```python
from build123d import *

# Parameters (mm, degrees)
SKETCH1_R               = 5.5
BOSS_EXTRUDE1_DEPTH     = 6
CUT_EXTRUDE1_DEPTH      = 3
CUT_EXTRUDE1_DEPTH_BACK = 3
SKETCH3_W               = 5
SKETCH3_H               = 0.446225232


with BuildPart() as part:
    # Sketch1 → Boss-Extrude1 (new body)
    with BuildSketch(Plane(origin=(0, 0, 0), x_dir=(1, 0, 0), z_dir=(0, 1, 0))):
        with Locations(Location((0, 0, 0), (0, 0, 270))):
            Circle(SKETCH1_R)
    extrude(amount=BOSS_EXTRUDE1_DEPTH)

    # Sketch3 → Cut-Extrude1 (cut, two sides: drawn at the far end of the back side and taken through both)
    with BuildSketch(Plane(origin=(0, 3, 3), x_dir=(1, 0, 0), z_dir=(0, 0.7071067811865464, 0.7071067811865488)).offset(-CUT_EXTRUDE1_DEPTH_BACK)):
        with Locations((0.083557951, 4.409395003)):
            Rectangle(SKETCH3_W, SKETCH3_H)
    extrude(amount=CUT_EXTRUDE1_DEPTH + CUT_EXTRUDE1_DEPTH_BACK, mode=Mode.SUBTRACT)


solid = part.part
```
Check sheet for the modelled part. Datum: model origin and axes. Units: mm. A direction names the side the tool comes from. Round coordinates to 2 decimals unless told otherwise and drop trailing zeros. Order: outer loops, then holes, each group sorted by start corner. A loop starts at its lowest first (then second) coordinate and runs counter-clockwise, first axis right, second up. Notation, with made-up numbers: M 50,45 L 65,45 A11 ccw 65,52 Z; hole C 62,-20 d2. An arc over 180 degrees is marked long. Answer in a Markdown table with one row per item.
(1) Gauge pin test, flat ends, axial feed: pin 1 (1.7 mm diameter, centred on y = 5, z = -1.5, fed in from +X); pin 2 (1 mm diameter, centred on x = -2, y = 3.5, fed in from +Z); pin 3 (1.5 mm diameter, centred on y = 5.5, z = 1.5, fed in from +X); pin 4 (1 mm diameter, centred on x = 0.5, z = -2, fed in from -Y). Record the tip position at first contact, or that the pin passes through.
Findings:
| item | result |
|---|---|
| pin 1 | stops at x = 5.46 |
| pin 2 | stops at z = 5.29 |
| pin 3 | stops at x = 5.45 |
| pin 4 | stops at y = 0 |
(2) Draft check along Y on faces 3 (the flat face through (2.584, 5.1, -1.2)), 4 (the cylindrical face through (-5.37, 2.96, -1.19)), 5 (the flat face through (0, 0, 0)). Enter one of: +Y half, -Y half, draft (parallel to the pull), parting line (faces both ways), or undercut.
Findings:
| item | result |
|---|---|
| face 3 | undercut |
| face 4 | draft |
| face 5 | -Y half |
(3) Section check C-C on y = 3.4. Record the boundary of the cut face in (x, z).
Findings:
| item | result |
|---|---|
| outline | C 0,0 d11 |
(4) Material ranges on line 1 along Y through (x, z) = (1.5, -0.75); line 2 along Z through (x, y) = (1.5, 5.15); line 3 along Z through (x, y) = (2, 4.55), recorded low to high. Write a range as from..to.
Findings:
| item | result |
|---|---|
| line 1 | y = 0..5.17, 5.8..6 |
| line 2 | z = -5.29..-1.4, -0.77..5.29 |
| line 3 | z = -5.12..-2, -1.37..5.12 |
(5) Section check B-B on z = -2.25. Record the boundary of the cut face in (x, y).
Findings:
| item | result |
|---|---|
| outline | M -5.02,0 L 5.02,0 L 5.02,6 L -5.02,6 Z; hole M -2.42,4.01 L 2.58,4.01 L 2.58,4.3 L -2.42,4.3 Z |
(6) Section check D-D on x = 1.75. Record the boundary of the cut face in (y, z).
Findings:
| item | result |
|---|---|
| outline | M 0,-5.21 L 6,-5.21 L 6,-0.55 L 4.15,-2.4 L 3.84,-2.08 L 6,0.08 L 6,5.21 L 0,5.21 Z |
(7) Section check A-A on x = 0. Record the boundary of the cut face in (y, z).
Findings:
| item | result |
|---|---|
| outline | M 0,-5.5 L 6,-5.5 L 6,-0.55 L 4.15,-2.4 L 3.84,-2.08 L 6,0.08 L 6,5.5 L 0,5.5 Z |
(8) Set-up check for faces 1 (the flat face through (0, 6, 1)), 2 (the flat face through (-2.416, 5.1, -1.2)): record each of +Z, -Z, +X, -X, +Y, -Y from which the full face is reachable in a straight line by a thin tool's end or side.
Findings:
| item | result |
|---|---|
| face 1 | +Z, -Z, +X, -X, +Y |
| face 2 | none |
